Input: part model. Units: mm. Frame: model coordinates. Face numbers are marked on the shaded views. A direction names the side the tool comes from. Coordinates: 2 decimals unless noted, no trailing zeros. Write each loop counter-clockwise with the first axis right and the second up, starting at its lowest first coordinate (ties: lowest second). Pieces come first, ordered by that corner, then holes. Notation, with made-up numbers: M 22,46 L 68,46 A25 cw 68,83 Z; hole C -26,-13.5 d4. An arc over 180 degrees is marked long. Use CSV: the item, a comma, the result in double quotes.
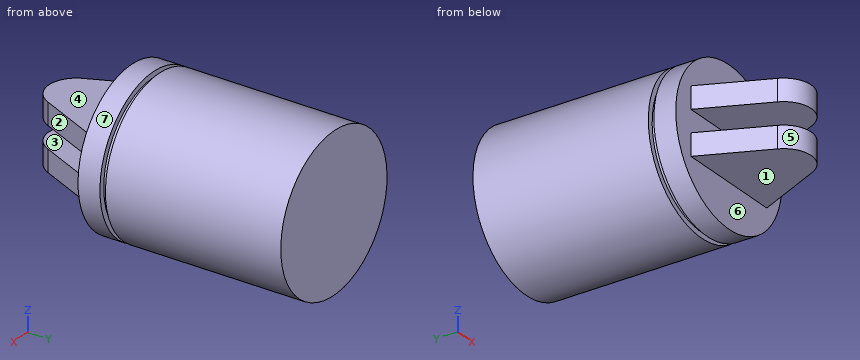
```python
from build123d import *

# Parameters (mm, degrees)
BOSS_EXTRUDE1_START = 5
BOSS_EXTRUDE1_DEPTH = 10
LPATTERN1_COUNT     = 2
LPATTERN1_PITCH     = 20
SKETCH2_R           = 35
SKETCH2_R_2         = 32.5
SKETCH2_W           = 50
SKETCH2_H           = 10
BOSS_EXTRUDE2_DEPTH = 10
BOSS_EXTRUDE3_START = 10
SKETCH2_3_R         = 32.5
BOSS_EXTRUDE3_DEPTH = 2.5
BOSS_EXTRUDE4_START = 12.5
SKETCH2_4_R         = 35
BOSS_EXTRUDE4_DEPTH = 80


with BuildPart() as part:
    # Sketch1 → Boss-Extrude1 (new body)
    with BuildSketch(Plane.XY.offset(BOSS_EXTRUDE1_START)):
        with BuildLine():
            Line((-11.392972847, -5.142972847), (-25, 25))
            Line((-25, 25), (25, 25))
            Line((25, 25), (11.392972847, -5.142972847))
            ThreePointArc((11.392972847, -5.142972847), (0, -12.5), (-11.392972847, -5.142972847))
        make_face()
    extrude(amount=BOSS_EXTRUDE1_DEPTH)


with BuildPart() as lpattern1_1:
    # LPattern1: pattern copy
    add(part.part.moved(Location(Vector(0, 0, -1) * (1 * LPATTERN1_PITCH))))


with BuildPart() as part_1:
    add(part.part)

    add(lpattern1_1.part)  # Boss-Extrude2 merges LPattern1_1
    # Sketch2 → Boss-Extrude2 (add)
    # profile 1 of 3: a face of its own
    with BuildSketch(Plane(origin=(0, 25, 0), x_dir=(1, 0, 0), z_dir=(0, 1, 0))):
        with Locations(Location((0, 0, 0), (0, 0, 270))):
            Circle(SKETCH2_R)
        Circle(SKETCH2_R_2, mode=Mode.SUBTRACT)
    # profile 2 of 3: a face of its own
    with BuildSketch(Plane(origin=(0, 25, 0), x_dir=(1, 0, 0), z_dir=(0, 1, 0))):
        Circle(SKETCH2_R_2)
        with Locations((0, -10)):
            Rectangle(SKETCH2_W, SKETCH2_H, mode=Mode.SUBTRACT)
    # profile 3 of 3: a face of its own
    with BuildSketch(Plane(origin=(0, 25, 0), x_dir=(1, 0, 0), z_dir=(0, 1, 0))):
        with Locations((0, -10)):
            Rectangle(SKETCH2_W, SKETCH2_H)
    extrude(amount=BOSS_EXTRUDE2_DEPTH)

    # Sketch2<3> → Boss-Extrude3 (add)
    with BuildSketch(Plane(origin=(0, 25, 0), x_dir=(1, 0, 0), z_dir=(0, 1, 0)).offset(BOSS_EXTRUDE3_START)):
        with Locations(Location((0, 0, 0), (0, 0, 270))):
            Circle(SKETCH2_3_R)
    extrude(amount=BOSS_EXTRUDE3_DEPTH)

    # Sketch2<4> → Boss-Extrude4 (add)
    with BuildSketch(Plane(origin=(0, 25, 0), x_dir=(1, 0, 0), z_dir=(0, 1, 0)).offset(BOSS_EXTRUDE4_START)):
        with Locations(Location((0, 0, 0), (0, 0, 270))):
            Circle(SKETCH2_4_R)
    extrude(amount=BOSS_EXTRUDE4_DEPTH)


solid = part_1.part
```
1. Material intervals for line 1 (Z direction, x = -11, y = 19); line 2 (Y direction, x = 15, z = 28); line 3 (Z direction, x = -14.5, y = 74), sorted ascending. Write a range as [from, to].
Resolved:
line 1,"z = [-15, -5], [5, 15]"
line 2,"y = [25, 117.5]"
line 3,"z = [-31.86, 31.86]"
2. Mould query, pull axis Z, two halves, no side actions, for the marked faces 5, 6 and 7. Classes: pulls with the +Z half, pulls with the -Z half, needs draft (parallel to the pull), parting line crosses it, or undercut.
Resolved:
face 5,"needs draft"
face 6,"undercut"
face 7,"parting line crosses it"
3. Section D-D (y = 89). Return loops of the section in (x, z).
Resolved:
outline,"C 0,0 d70"
4. Access query for the marked faces 1, 2, 3 and 4. Directions: +Z, -Z, +X, -X, +Y, -Y. A direction counts if a zero-diameter tool reaches every point of the face in a straight line with its end or side. Return the directions, or none.
Resolved:
face 1,"-Z, +X, -X, -Y"
face 2,"+Z, -Z, +X, -Y"
face 3,"+X, -X, -Y"
face 4,"+Z, +X, -X, -Y"
5. Contact query for flat-ended pins moving along their axis: pin 1 Ø1 at (x, y) = (-13.5, 17.5) entering from +Z; pin 2 Ø10 at (x, z) = (-9.5, -5.5) entering from -Y; pin 3 Ø4 at (x, y) = (-8.5, 45) entering from -Z; pin 4 Ø2 at (x, y) = (0.5, 54.5) entering from -Z. Output: stop coordinate, or through.
Resolved:
pin 1,"stops at z = 15"
pin 2,"stops at y = -11.66"
pin 3,"stops at z = -34.39"
pin 4,"stops at z = -35"
6. Section C-C (x = 0). Return loops of the section in (y, z).
Resolved:
outline,"M -12.5,-15 L 25,-15 L 25,-35 L 35,-35 L 35,-32.5 L 37.5,-32.5 L 37.5,-35 L 117.5,-35 L 117.5,35 L 37.5,35 L 37.5,32.5 L 35,32.5 L 35,35 L 25,35 L 25,15 L -12.5,15 L -12.5,5 L 25,5 L 25,-5 L -12.5,-5 Z"
7. Section B-B (z = 0). Return loops of the section in (x, y), then the cut area to 3 significant figures.
Resolved:
outline,"M -35,25 L 35,25 L 35,35 L 32.5,35 L 32.5,37.5 L 35,37.5 L 35,117.5 L -35,117.5 L -35,37.5 L -32.5,37.5 L -32.5,35 L -35,35 Z"
area,"6,460 mm^2"
8. Section A-A (y = 21). Return loops of the section in (x, z).
Resolved:
outline,"M -23.19,-15 L 23.19,-15 L 23.19,-5 L -23.19,-5 Z; M -23.19,5 L 23.19,5 L 23.19,15 L -23.19,15 Z"
